Geometry check sheet. Reference: the model listing, model coordinates, mm. A direction names the side the tool comes from. Give positions to 0.01 mm unless a question says otherwise; leave off trailing zeros. Write each loop counter-clockwise with the first axis right and the second up, starting at its lowest first coordinate (ties: lowest second). Pieces come first, ordered by that corner, then holes. Notation, with made-up numbers: M 8,20.25 L 36,20.25 A27 cw 36,36.25 Z; hole C -36.5,38 d6. An arc over 180 degrees is marked long. One line per item, written item: value. Start each with the question number.
1. Tool access check on faces 4 (the face through (22, 2.034, 1)), 5 (the face through (30, 20.134, 1)), 6 (the face through (28, 9, 0)). Record the directions out of +Z, -Z, +X, -X, +Y, -Y that give a thin tool (end or side, any length) a straight path to the whole face; none if there is none.
2. Cross-section at C-C on x = 13. Record the cut outline in (y, z).
3. Cross-section at B-B on x = 29.75. Record the cut outline in (y, z).
4. Scan lines: line 1 (Y direction, x = 29.75, z = 1.45); line 2 (Y direction, x = 0, z = 1.3); line 3 (Y direction, x = 20, z = 2.4). Record each from-to range of solid material in increasing order.
5. Gauge pin test, flat ends, axial feed: pin 1 (1.5 mm diameter, centred on x = 12.5, z = 2, fed in from +Y); pin 2 (0.9 mm diameter, centred on x = 23, z = 2, fed in from -Y). Record the tip position at first contact, or that the pin passes through.
6. Cross-section at D-D on z = 1.5. Count the separate pieces of the cut face and the enclosed holes in it, then the cut area to 3 significant figures.
7. Release check for a two-part mould opening along Y. For faces 1 (the face through (47.65, 8, 1)), 2 (the face through (25.1, 8, 1)), 3 (the face through (13.5, 20.9, 1.5)) record: pulls with the +Y half, pulls with the -Y half, needs draft (parallel to the pull), parting line crosses it, or undercut.
8. Cross-section at A-A on y = 10.25. Record the cut outline in (x, z), then the cut area to 4 significant figures.
from build123d import *

# Parameters (mm, degrees)
SKETCH1_R           = 1.5
BOSS_EXTRUDE1_DEPTH = 3


with BuildPart() as part:
    # Sketch1 → Boss-Extrude1 (new body)
    with BuildSketch(Plane.XY):
        with BuildLine():
            Line((44.671696982, 20.134210536), (14.948744814, 20.134210536))
            ThreePointArc((14.948744814, 20.134210536), (13.508437041, 20.900264991), (12.086852766, 20.1))
            Line((12.086852766, 20.1), (0.079653818, 19.618721067))
            ThreePointArc((0.079653818, 19.618721067), (-1.951692295, 18.711836018), (-2.8, 16.655338617))
            Line((-2.8, 16.655338617), (-2.8, 0.013082454))
            ThreePointArc((-2.8, 0.013082454), (-1.91420574, -2.147770093), (0.252672107, -3.018721067))
            Line((0.252672107, -3.018721067), (12.259871055, -3.5))
            ThreePointArc((12.259871055, -3.5), (13.584562431, -4.127366103), (14.862137332, -3.408897008))
            Line((14.862137332, -3.408897008), (44.5850895, -3.408897008))
            ThreePointArc((44.5850895, -3.408897008), (46.728413048, -2.573492827), (47.65, -0.465789464))
            Line((47.65, -0.465789464), (47.65, 17.134210536))
            ThreePointArc((47.65, 17.134210536), (46.779005205, 19.247896538), (44.671696982, 20.134210536))
        make_face()
        with Locations((29.75, 17.026583922)):
            Circle(SKETCH1_R, mode=Mode.SUBTRACT)
        with Locations((44.65, 17.334210536)):
            Circle(SKETCH1_R, mode=Mode.SUBTRACT)
        with Locations((44.65, -0.665789465)):
            Circle(SKETCH1_R, mode=Mode.SUBTRACT)
        with Locations((29.75, 0.383476379)):
            Circle(SKETCH1_R, mode=Mode.SUBTRACT)
        Circle(SKETCH1_R, mode=Mode.SUBTRACT)
        with Locations((0, 16.787592152)):
            Circle(SKETCH1_R, mode=Mode.SUBTRACT)
        Polygon((4.75, 14.634210535), (1.9, 14.634210535), (1.9, 2.034210535), (7.65, 2.034210535), (7.65, -0.865789465), (19.65, -0.865789465), (19.65, 2.034210535), (25.1, 2.034210535), (25.1, 14.634210535), (22.25, 14.634210535), (22.25, 17.634210536), (4.75, 17.634210536), align=None, mode=Mode.SUBTRACT)
    extrude(amount=BOSS_EXTRUDE1_DEPTH)


solid = part.part
Report:
1. face 4: +Z, -Z
1. face 5: +Z, -Z, +X, +Y
1. face 6: -Z, +X, -X, +Y, -Y
2. outline: M -4.04,0 L -0.87,0 L -0.87,3 L -4.04,3 Z; M 17.63,0 L 20.82,0 L 20.82,3 L 17.63,3 Z
3. outline: M -3.41,0 L -1.12,0 L -1.12,3 L -3.41,3 Z; M 1.88,0 L 15.53,0 L 15.53,3 L 1.88,3 Z; M 18.53,0 L 20.13,0 L 20.13,3 L 18.53,3 Z
4. line 1: y = -3.41 to -1.12, 1.88 to 15.53, 18.53 to 20.13
4. line 2: y = -3.01 to -1.5, 1.5 to 15.29, 18.29 to 19.61
4. line 3: y = -3.41 to 2.03, 17.63 to 20.13
5. pin 1: stops at y = 20.88
5. pin 2: stops at y = -3.41
6. separate pieces: 1
6. enclosed holes: 7
6. area: 753 mm^2
7. face 1: needs draft
7. face 2: undercut
7. face 3: pulls with the +Y half
8. outline: M -2.8,0 L 1.9,0 L 1.9,3 L -2.8,3 Z; M 25.1,0 L 47.65,0 L 47.65,3 L 25.1,3 Z
8. area: 81.75 mm^2
